Autodesk Inventor part; units mm, degrees
ref_plane "YZ Plane" through (0, 0, 0) normal (1, 0, 0) x (0, 1, 0)
ref_plane "XZ Plane" through (0, 0, 0) normal (0, 1, 0) x (-1, 0, 0)
ref_plane "XY Plane" through (0, 0, 0) normal (0, 0, 1) x (1, 0, 0)
sketch "Sketch1" plane through (0, 0, 0) normal (1, 0, 0) x (0, 1, 0)
  line L0 (0, 0) -> (63.5, 0)
  line L1 (63.5, 0) -> (63.5, -149.225)
  line L2 (63.5, -149.225) -> (12.7, -149.225)
  circle A0 centre (-31.75, -53.975) radius 14.2875
  line L3 (63.5, -25.4) -> (-43.502, -25.4) construction
  circle A1 centre (50.8, -12.7) radius 3.175
  circle A2 centre (-104.775, -12.7) radius 3.175
  line L4 (12.7, -149.225) -> (-114.3, -69.85)
  line L5 (-114.3, -69.85) -> (-114.3, 0)
  line L6 (-114.3, 0) -> (0, 0) construction
  circle A3 centre (-85.725, -53.975) radius 14.2875
  line L7 (-53.2384, 0) -> (-95.25, 0)
  line L8 (-95.25, 0) -> (-95.25, 45.1866) construction
  line L9 (-95.25, 45.1866) -> (-53.2384, 45.1866) construction
  line L10 (-53.2384, 45.1866) -> (-53.2384, 0) construction
  line L11 (-95.25, 45.1866) -> (-114.3, 0) construction
  line L12 (-53.2384, 45.1866) -> (0, 0) construction
  circle A4 centre (-56.3011, 6.2145) radius 2.3813
  circle A5 centre (-92.2105, 42.1471) radius 2.3813
  line L13 (0, 0) -> (-49.0855, 50.8)
  line L14 (-49.0855, 50.8) -> (-99.8855, 50.8)
  line L15 (-99.8855, 50.8) -> (-114.3, 0)
  circle A6 centre (-74.2558, 24.1808) radius 7.9375
  line L16 (-92.2105, 42.1471) -> (-74.2558, 24.1808) construction
  line L17 (-74.2558, 24.1808) -> (-56.3011, 6.2145) construction
  circle A7 centre (38.1, -127) radius 14.2875
  circle A8 centre (22.225, -88.9) radius 3.175
  circle A9 centre (50.8, -63.5) radius 3.175
  circle A10 centre (25.4, -38.1) radius 3.175
  circle A11 centre (-79.375, -12.7) radius 3.175
  dimension "d1" = 28.575
  dimension "d2" = 63.5
  dimension "d6" = 25.4
  dimension "d7" = 6.35
  dimension "d8" = 6.35
  dimension "d9" = 12.7
  dimension "d10" = 12.7
  dimension "d12" = 12.7
  dimension "d17" = 50.8
  dimension "d18" = 114.3
  dimension "d19" = 9.525
  dimension "d20" = 53.975
  dimension "d21" = 28.575
  dimension "d24" = 53.975
  dimension "d25" = 69.85
  dimension "d26" = 53.975
  dimension "d27" = 149.225
  dimension "d28" = 107.002
  dimension "d29" = 42.0116
  dimension "d30" = 19.05
  dimension "d31" = 45.1866
  dimension "d32" = 50.8
  dimension "d33" = 4.7625
  dimension "d34" = 3.0395
  dimension "d35" = 3.0395
  dimension "d36" = 6.2145
  dimension "d37" = 50.8
  dimension "d38" = 50.8
  dimension "d39" = 4.1529
  dimension "d40" = 15.875
  dimension "d42" = 22.225
  dimension "d43" = 25.4
  dimension "d44" = 28.575
  dimension "d45" = 6.35
  dimension "d46" = 6.35
  dimension "d47" = 6.35
  dimension "d48" = 38.1
  dimension "d49" = 38.1
  dimension "d50" = 41.275
  dimension "d51" = 12.7
  dimension "d52" = 63.5
  dimension "d53" = 88.9
  dimension "d54" = 6.35
  dimension "d55" = 12.7
  dimension "d56" = 25.4
extrude "Extrusion1" add sketch "Sketch1" along normal blind 6.35 contours L0 L1 L2 L4 L5 L15 L14 L13 | A3 | A4 | A5 | A6 | A7 | A8 | A9 | A10 | A11
extrude "Extrusion2" cut sketch "Sketch1" along normal blind 25.4 contours A3 | A4 | A5 | A6 | A7 | A8 | A9 | A10 | A11
equation "\"BendRadius\" = Thickness"
equation "\"BendReliefWidth\" = Thickness"
equation "\"BendReliefDepth\" = 0.5 * Thickness"
equation "\"CornerReliefSize\" = 4 * Thickness"
equation "\"MinimumRemnant\" = 2 * Thickness"
equation "\"TransitionRadius\" = BendRadius"
equation "\"JacobiRadiusSize\" = Thickness"
equation "\"GapSize\" = Thickness"
properties part number "15102898-16-P-0302" material "Aluminum 6061"
Build history of the part. All positions in model axes, mm. A direction names the side the tool comes from. Give positions to 0.01 mm unless a question says otherwise; leave off trailing zeros. Order: outer loops, then holes, each group sorted by start corner. A loop starts at its lowest first (then second) coordinate and runs counter-clockwise, first axis right, second up. Notation, with made-up numbers: M 56,-6 L 66,-6 A14 cw 66,3 Z; hole C 74.5,35 d4. An arc over 180 degrees is marked long. Put each result on its own line as item: value.
Item 1: Flat gauge pins, fed straight in: pin 1 Ø1 at (x, z) = (1, 6.5) entering from +Y; pin 2 Ø1.5 at (x, z) = (1, -93.5) entering from -Y. Where does each tip first touch, or does it go through?
From the geometry:
pin 1: stops at y = -5.8
pin 2: stops at y = -77.66
Item 2: Slice it at B-B, the plane y = -30.5. Write the cut outline in (x, z) (3 decimals), plus the area to 3 significant figures.
From the geometry:
outline: M 0,-122.225 L 6.35,-122.225 L 6.35,-68.208 L 0,-68.208 Z; M 0,-39.742 L 6.35,-39.742 L 6.35,31.565 L 0,31.565 Z
area: 796 mm2
Item 3: Probe line 1 (Y direction, x = 4.5, z = -38.1) (3 decimals); line 2 (Y direction, x = 5, z = -63.5) (3 decimals); line 3 (Z direction, x = 3.75, y = 50.8) (3 decimals). List the from-to ranges inside material, lowest first. Write a range as [from, to].
From the geometry:
line 1: y = [-114.3, 22.225], [28.575, 63.5]
line 2: y = [-114.3, -96.374], [-75.076, -42.399], [-21.101, 47.625], [53.975, 63.5]
line 3: z = [-149.225, -133.545], [-120.455, -66.675], [-60.325, -15.875], [-9.525, 0]
Item 4: Slice it at C-C, the plane z = -12.7. Write the cut outline in (x, y) (3 decimals).
From the geometry:
outline: M 0,-114.3 L 6.35,-114.3 L 6.35,-107.95 L 0,-107.95 Z; M 0,-101.6 L 6.35,-101.6 L 6.35,-82.55 L 0,-82.55 Z; M 0,-76.2 L 6.35,-76.2 L 6.35,47.625 L 0,47.625 Z; M 0,53.975 L 6.35,53.975 L 6.35,63.5 L 0,63.5 Z
Item 5: Two-plate mould, pull along Z, no slides. Class faces 3 (the cylindrical face through (3.131, -66.924, 27.221)), 4 (the flat face through (3, 63.5, -74)), 5 (the flat face through (3, -74, 50.8)): +Z half, -Z half, draft (parallel to the pull), parting line (faces both ways), or undercut.
From the geometry:
face 3: undercut
face 4: draft
face 5: +Z half
Item 6: Slice it at D-D, the plane x = 3.75. Give the number of separate pieces and of enclosed holes in the cut face, plus the area to 3 significant figures.
From the geometry:
separate pieces: 1
enclosed holes: 12
area: 23,300 mm2
Item 7: 3-axis set-ups, long thin cutter, end or side, ignore diameter. For faces 1 (the cylindrical face through (3.131, -76.347, -13.654)), 2 (the flat face through (3, 31, 0)): which of +Z, -Z, +X, -X, +Y, -Y reach the whole face in a straight line?
From the geometry:
face 1: +X, -X
face 2: +Z, +X, -X, +Y
Item 8: Slice it at A-A, the plane z = -127. Write the cut outline in (x, y), plus the area to 3 significant figures.
From the geometry:
outline: M 0,-22.86 L 6.35,-22.86 L 6.35,23.81 L 0,23.81 Z; M 0,52.39 L 6.35,52.39 L 6.35,63.5 L 0,63.5 Z
area: 367 mm2
